from build123d import *

# Parameters (mm, degrees)
F0_R     = 15.5
F1_DEPTH = 5
F2_SIZE2 = 4.99999
F2_SIZE  = 0.99999
F3_W     = 10
F3_H     = 2
F4_DEPTH = 2


# Not quite as in the source:
# - a fillet or chamfer is up to 0.001 mm smaller than in the source, because OpenCascade refuses the exact size


with BuildPart() as f1:
    # F0 (on Top) → F1 (new body)
    with BuildSketch(Plane.XY):
        Circle(F0_R)
    extrude(amount=F1_DEPTH)

    # F2 (size 1 and 5 in the source; OpenCascade refuses exactly that, so slightly less here)
    f2_edges = [f1.edges().sort_by_distance(p)[0] for p in [
        (-15.5, 0, 5),
    ]]
    f2_side = f1.faces().sort_by_distance((0, 0, 5))[0]
    chamfer(f2_edges, length=F2_SIZE, length2=F2_SIZE2, reference=f2_side)

    # F3 (on face) → F4 (cut)
    with BuildSketch(Plane(origin=(0, 0, 0), x_dir=(1, 0, 0), z_dir=(0, 0, -1))):
        with Locations((0.2559603993, -0.1766888017)):
            Rectangle(F3_W, F3_H)
    extrude(amount=-F4_DEPTH, mode=Mode.SUBTRACT)


solid = f1.part
Read the model definition and answer for the solid it produces. Units are mm, in the model's axes. A direction names the side the tool comes from. Give positions to 0.01 mm unless a question says otherwise; leave off trailing zeros. Loops run counter-clockwise (first coordinate to the right, second up) from the corner with the lowest first, then second, coordinate; pieces in that order, holes last. Notation, with made-up numbers: (0.25, 1) -> (22.25, 1) arc R24 cw to (22.25, 20) -> close; hole circle Ø4 at (3.5, 43). An arc over 180 degrees is marked (long way). Answer as CSV lines item,"result".
Item 1: Each of these flat-tipped pins is pushed along its axis until it touches: pin 1 (3 mm diameter, centred on x = -10.5, z = 2.5, fed in from +Y); pin 2 (2 mm diameter, centred on y = 0.5, z = 1.5, fed in from +X); pin 3 (1.5 mm diameter, centred on x = -9.5, z = 2, fed in from -Y); pin 4 (2 mm diameter, centred on x = -2, y = 0, fed in from -Z). Where does it stop, or does it pass through?
Returned:
pin 1,"stops at y = 12.06"
pin 2,"stops at x = 15.39"
pin 3,"stops at y = -12.34"
pin 4,"stops at z = 0"
Item 2: Determine the mould class of faces 1 (the face through (5.256, 0, 1)), 2 (the face through (0, 0, 5)), 3 (the face through (-3.157, -14.216, 4.687)) for opening direction X: +X half, -X half, draft (parallel to the pull), parting line (faces both ways), or undercut.
Returned:
face 1,"undercut"
face 2,"draft"
face 3,"parting line"
Item 3: Find section A-A on z = 1.2. Give the vertices of the cut face in (x, y), plus the area to 3 significant figures.
Returned:
outline,"circle Ø30.52 at (0, 0); hole (-4.74, -0.82) -> (5.26, -0.82) -> (5.26, 1.18) -> (-4.74, 1.18) -> close"
area,"712 mm²"
Item 4: Consider line 1 (Y direction, x = -0.5, z = 1.85); line 2 (Y direction, x = -1.5, z = 0.5); line 3 (X direction, y = 2, z = 4.4). Determine where each line is inside the solid, lowest interval first. Write a range as [from, to].
Returned:
line 1,"y = [-15.12, -0.82], [1.18, 15.12]"
line 2,"y = [-15.33, -0.82], [1.18, 15.33]"
line 3,"x = [-14.48, 14.48]"
Item 5: Find section D-D on z = 2.8. Give the vertices of the cut face in (x, y), plus the area to 3 significant figures.
Returned:
outline,"circle Ø29.88 at (0, 0)"
area,"701 mm²"
Item 6: For faces 4 (the face through (0, -0.823, 1)), 5 (the face through (0, -3, 0)), determine the directions among +Z, -Z, +X, -X, +Y, -Y from which every point of the face is accessible in a straight line to the end or side of a thin tool.
Returned:
face 4,"-Z"
face 5,"-Z, +X, -X, +Y, -Y"
